Can you work these out from the model? Positions are in its coordinate system, mm. A direction names the side the tool comes from. Coordinates: 2 decimals unless noted, no trailing zeros. Loops run counter-clockwise (first coordinate to the right, second up) from the corner with the lowest first, then second, coordinate; pieces in that order, holes last. Notation, with made-up numbers: M 89,28 L 93,28 A14 cw 93,52 Z; hole C -28.5,19.25 d8. An arc over 180 degrees is marked long. Return JSON: item names as keys, results as strings. Group by question number.
```python
from build123d import *

# Parameters (mm, degrees)
SKETCH_1_R      = 3
EXTRUDE_1_DEPTH = 8
EXTRUDE_START   = -4
EXTRUDE_3_DEPTH = 3.5


with BuildPart() as part:
    # 草图1 → 凸台-拉伸1 (new body)
    with BuildSketch(Plane(origin=(0, 0, 0), x_dir=(1, 0, 0), z_dir=(0, 1, 0))):
        Polygon((0, 0), (0, 64), (-4.185096591, 64), (-4.185096591, 33.185096591), (-33.185096591, 4.185096591), (-64, 4.185096591), (-64, 0), align=None)
        with Locations(Location((-15.385096591, 15.385096591, 0), (0, 0, 270))):
            Circle(SKETCH_1_R, mode=Mode.SUBTRACT)
    extrude(amount=EXTRUDE_1_DEPTH)

    # 草图4 → 凸台-拉伸3 (add, symmetric)
    with BuildSketch(Plane.XZ.offset(EXTRUDE_START)):
        Polygon((-6.385096591, -30.985096591), (-6.385096591, -64), (-4.185096591, -64), (-4.185096591, -33.185096591), align=None)
        Polygon((-64, -4.185096591), (-64, -6.385096591), (-30.985096591, -6.385096591), (-33.185096591, -4.185096591), align=None)
    extrude(amount=EXTRUDE_3_DEPTH, both=True)


solid = part.part
```
1) If we mould it in two halves opening along X, with no side actions, what happens to faces 6 (the face through (-6.385, 4, -47)), 7 (the face through (-5, 0.5, -47)), 8 (the face through (-13.36, 3.94, -17.6)), 9 (the face through (0, 4, -32))? For each: +X half, -X half, draft (parallel to the pull), parting line (faces both ways), or undercut.
2) Suppose I cut it at B-B, the plane z = -14. List the corners of the cut face in (x, y) for me.
3) For pin 1 (2.5 mm diameter, centred on x = -42.5, z = -6, fed in from +Y); pin 2 (0.6 mm diameter, centred on y = 7.5, z = -43.5, fed in from -X); pin 3 (1.1 mm diameter, centred on x = -47, z = -5, fed in from -Y), each with a flat end and sliding along its axis, tell me the tip position at first contact or that it passes through.
4) Suppose I cut it at A-A, the plane x = -39. List the corners of the cut face in (y, z) for me.
5) For faces 1 (the face through (-48, 4, -6.385)), 2 (the face through (-48, 0.5, -5)), 3 (the face through (-48, 7.5, -5)), 4 (the face through (-64, 4, -3)), 5 (the face through (-18, 8, -13)), which set-ups out of +Z, -Z, +X, -X, +Y, -Y let a thin tool reach every point of the face, with its end or its side?
6) If I drill on line 1 (Z direction, x = -39, y = 1.75); line 2 (Z direction, x = -17, y = 2.25), over which ranges is the centre line in solid material (lowest first)? Write a range as from..to.
7) Suppose I cut it at C-C, the plane z = -51. List the corners of the cut face in (x, y) for me, then the cut area to 3 significant figures.
8) Suppose I cut it at D-D, the plane x = -13.5. List the corners of the cut face in (y, z) for me.
Returned:
{
 "1": {"face 6": "-X half", "face 7": "draft", "face 8": "undercut", "face 9": "+X half"},
 "2": {"outline": "M -23.37,0 L -18.05,0 L -18.05,8 L -23.37,8 Z; M -12.72,0 L 0,0 L 0,8 L -12.72,8 Z"},
 "3": {"pin 1": "stops at y = 7.5", "pin 2": "stops at x = -6.39", "pin 3": "stops at y = 0.5"},
 "4": {"outline": "M 0,-4.19 L 0.5,-4.19 L 0.5,-6.39 L 7.5,-6.39 L 7.5,-4.19 L 8,-4.19 L 8,0 L 0,0 Z"},
 "5": {"face 1": "-Z, -X, +Y, -Y", "face 2": "-Z, -X, -Y", "face 3": "-Z, -X, +Y", "face 4": "+Z, -Z, -X, +Y, -Y", "face 5": "+Z, -Z, +X, -X, +Y"},
 "6": {"line 1": "z = -6.39..0", "line 2": "z = -20.37..-17.91, -12.86..0"},
 "7": {"outline": "M -6.39,0.5 L -4.19,0.5 L -4.19,0 L 0,0 L 0,8 L -4.19,8 L -4.19,7.5 L -6.39,7.5 Z", "area": "48.9 mm²"},
 "8": {"outline": "M 0,-23.87 L 8,-23.87 L 8,-17.72 L 0,-17.72 Z; M 0,-13.05 L 8,-13.05 L 8,0 L 0,0 Z"}
}
